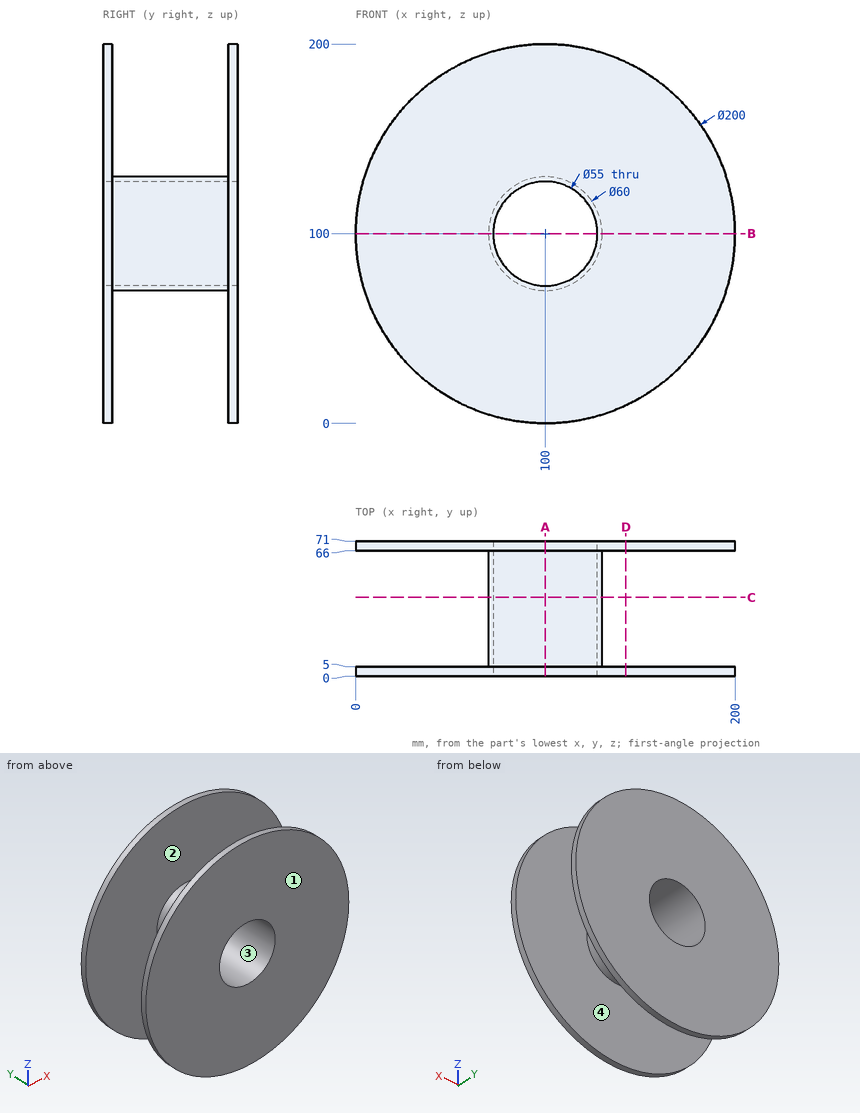
Check sheet for the drawn part. Datum: minimum x, y, z corner. Units: mm. A direction names the side the tool comes from. Round coordinates to 2 decimals unless told otherwise and drop trailing zeros. Write each loop counter-clockwise with the first axis right and the second up, starting at its lowest first coordinate (ties: lowest second). Pieces come first, ordered by that corner, then holes. Notation, with made-up numbers: (73.5, 72.5) - (101.5, 72.5) arc R16 ccw to (101.5, 96.5) - close; hole circle Ø6 at (-15, 61). An arc over 180 degrees is marked (long way). Return JSON: item names as keys, results as strings.
Q1. Cross-section at B-B (z = 100). Record the boundary of the cut face in (x, y).
Returned:
{"outline": "(0, 0) - (72.5, 0) - (72.5, 71) - (0, 71) - (0, 66) - (70, 66) - (70, 5) - (0, 5) - close; (127.5, 0) - (200, 0) - (200, 5) - (130, 5) - (130, 66) - (200, 66) - (200, 71) - (127.5, 71) - close"}
Q2. Scan lines: L1, parallel to Z at x = 100, y = 30; L2, parallel to Y at x = 118, z = 74.5; L3, parallel to X at y = 27.5, z = 85.5. Record each from-to range of solid material in increasing order. Write a range as from..to.
Returned:
{"L1": "z = 70..72.5, 127.5..130", "L2": "y = 0..5, 66..71", "L3": "x = 73.74..76.63, 123.37..126.26"}
Q3. Access from +Z, -Z, +X, -X, +Y, -Y to the whole of each face (thin tool, end or side, straight path). Record for the marked faces 1 and 2.
Returned:
{"face 1": "+Z, -Z, +X, -X, -Y", "face 2": "none"}
Q4. Cross-section at C-C (y = 41.5). Record the boundary of the cut face in (x, z).
Returned:
{"outline": "circle Ø60 at (100, 100); hole circle Ø55 at (100, 100)"}
Q5. Cross-section at D-D (x = 142.5). Record the boundary of the cut face in (y, z).
Returned:
{"outline": "(0, 9.48) - (5, 9.48) - (5, 190.52) - (0, 190.52) - close; (66, 9.48) - (71, 9.48) - (71, 190.52) - (66, 190.52) - close"}
Q6. Depth check by flat-ended pin: P1, Ø3, axis at x = 99, y = 46, coming from the +Z side; P2, Ø3, axis at y = 30, z = 118, coming from the +X side; P3, Ø10, axis at x = 67.5, y = 44, coming from the -Z side. Enter the tip coordinate at first touch or a pass-through.
Returned:
{"P1": "stops at z = 130", "P2": "stops at x = 125.05", "P3": "stops at z = 88.01"}
Q7. Cross-section at A-A (x = 100). Record the boundary of the cut face in (y, z).
Returned:
{"outline": "(0, 0) - (5, 0) - (5, 70) - (66, 70) - (66, 0) - (71, 0) - (71, 72.5) - (0, 72.5) - close; (0, 127.5) - (71, 127.5) - (71, 200) - (66, 200) - (66, 130) - (5, 130) - (5, 200) - (0, 200) - close"}
Q8. Draft check along X on the marked faces 3 and 4. Enter one of: released by +X, released by -X, zero draft, split by the parting line, or undercut.
Returned:
{"face 3": "undercut", "face 4": "zero draft"}
